Can you work these out from the model? Positions are in its coordinate system, mm. Face numbers are marked on the shaded views. Round coordinates to 2 decimals unless told otherwise and drop trailing zeros. Order: outer loops, then holes, each group sorted by start corner. A loop starts at its lowest first (then second) coordinate and runs counter-clockwise, first axis right, second up. Notation, with made-up numbers: (68, 64.25) -> (120, 64.25) arc R23 cw to (120, 95.25) -> close; hole circle Ø4 at (38, 32.5). An arc over 180 degrees is marked (long way). Use a Markdown table: item, result. Add a question column.
Q1. If we section it at A-A on y = 40: List the corners of the cut face in (x, z) for me, plus the area to 3 significant figures.
Q2. I'm going to push flat-ended pins straight in: pin 1 Ø12 at (x, z) = (197.5, 69.5) entering from -Y; pin 2 Ø1 at (x, y) = (81, 61.5) entering from +Z; pin 3 Ø1 at (x, y) = (48.5, 67) entering from -Z. Where does each tip first touch, or does it pass through?
Q3. If we section it at D-D on z = 28.5: List the corners of the cut face in (x, y) for me, plus the area to 3 significant figures.
Q4. I need wall thicknesses on line 1 along X through (y, z) = (40, 71); line 2 along Y through (x, z) = (158, 40); line 3 along Y through (x, z) = (114, 69.5). Which ranges of each line are inside material? Lowest first, please. Write a range as [from, to].
Q5. If we section it at B-B on x = 168: List the corners of the cut face in (y, z) for me, plus the area to 3 significant figures.
Q6. We'd pull the mould along Y, two halves only. Please class the marked faces 1, 2 and 3: +Y half, -Y half, draft (parallel to the pull), parting line (faces both ways), or undercut.
Q7. If we section it at C-C on z = 6: List the corners of the cut face in (x, y) for me.
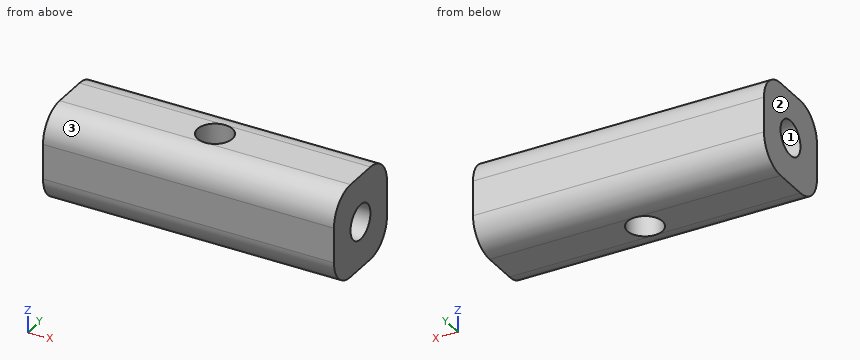
```python
from build123d import *

# Parameters (mm, degrees)
ESQUISSE1_W             = 250
ESQUISSE1_H             = 80
BOSS_EXTRU_1_DEPTH      = 80
ESQUISSE2_R             = 15
ENL_V_MAT_EXTRU_1_DEPTH = 275.40845468
ESQUISSE3_R             = 15
ENL_V_MAT_EXTRU_2_DEPTH = 80
CONG_1_R                = 25


with BuildPart() as part:
    # Esquisse1 → Boss.-Extru.1 (new body)
    with BuildSketch(Plane.XY):
        with Locations((125, 40)):
            Rectangle(ESQUISSE1_W, ESQUISSE1_H)
    extrude(amount=BOSS_EXTRU_1_DEPTH)

    # Esquisse2 → Enlèv. mat.-Extru.1 (cut, through all)
    with BuildSketch(Plane(origin=(250, 0, 0), x_dir=(0, 0, -1), z_dir=(1, 0, 0))):
        with Locations((-40, 40)):
            Circle(ESQUISSE2_R)
    extrude(amount=-ENL_V_MAT_EXTRU_1_DEPTH, mode=Mode.SUBTRACT)

    # Esquisse3 → Enlèv. mat.-Extru.2 (cut)
    with BuildSketch(Plane.XY.offset(80)):
        with Locations((125, 40)):
            Circle(ESQUISSE3_R)
    extrude(amount=-ENL_V_MAT_EXTRU_2_DEPTH, mode=Mode.SUBTRACT)

    # Congé1
    cong_1_edges = [part.edges().sort_by_distance(p)[0] for p in [
        (125, 80, 80),
        (125, 80, 0),
        (125, 0, 0),
        (125, 0, 80),
    ]]
    fillet(cong_1_edges, radius=CONG_1_R - 0.0001)  # a hair under: the kernel refuses the full size


solid = part.part
```
Answer below:
| question | item | result |
|---|---|---|
| 1 | outline | (0, 0) -> (110, 0) -> (110, 25) -> (0, 25) -> close; (0, 55) -> (110, 55) -> (110, 80) -> (0, 80) -> close; (140, 0) -> (250, 0) -> (250, 25) -> (140, 25) -> close; (140, 55) -> (250, 55) -> (250, 80) -> (140, 80) -> close |
| 1 | area | 11,000 mm² |
| 2 | pin 1 | y = 1.49 |
| 2 | pin 2 | z = 79.27 |
| 2 | pin 3 | z = 2.8 |
| 3 | outline | (0, 0) -> (250, 0) -> (250, 30.37) -> (136.5, 30.37) arc R15 cw to (113.5, 30.37) -> (0, 30.37) -> close; (0, 49.63) -> (113.5, 49.63) arc R15 cw to (136.5, 49.63) -> (250, 49.63) -> (250, 80) -> (0, 80) -> close |
| 3 | area | 15,000 mm² |
| 4 | line 1 | [0, 110], [140, 250] |
| 4 | line 2 | [0, 25], [55, 80] |
| 4 | line 3 | [4.63, 29.8], [50.2, 75.37] |
| 5 | outline | (0, 25) arc R25 ccw to (25, 0) -> (55, 0) arc R25 ccw to (80, 25) -> (80, 55) arc R25 ccw to (55, 80) -> (25, 80) arc R25 ccw to (0, 55) -> close; hole circle Ø30 at (40, 40) |
| 5 | area | 5,160 mm² |
| 6 | face 1 | undercut |
| 6 | face 2 | draft |
| 6 | face 3 | -Y half |
| 7 | outline | (0, 8.75) -> (250, 8.75) -> (250, 71.25) -> (0, 71.25) -> close; hole circle Ø30 at (125, 40) |
